from build123d import *

# Parameters (mm, degrees)
SKETCH1_W             = 2
SKETCH1_H             = 2
SKETCH1_W_2           = 21
SKETCH1_H_2           = 15
SKETCH1_H_3           = 1
IMU_BASE_DEPTH        = 7
SCREW_CHANNELS_DEPTH  = 14
SKETCH1_13_W          = 2
SKETCH1_13_H          = 1
NUT_CHANNELS_DEPTH    = 3
SKETCH2_W             = 23
SKETCH2_H             = 15
SOLDER_CHANNELS_DEPTH = 2.5
IMU_EXTENSION_DEPTH   = 15


with BuildPart() as part:
    # Sketch1 → IMU_Base (new body)
    with BuildSketch(Plane.XY):
        Polygon((-2, 0), (0, 0), (0, 1), (0, 5), (0, 6), (0, 21), (0, 21.55806344), (0, 22), (0, 26), (0, 27), (0.75, 27), (5.75, 27), (6.5, 27), (14.5, 27), (15.25, 27), (20.25, 27), (21, 27), (23, 27), (23, 29), (-2, 29), align=None)
        Polygon((0.75, 0), (0, 0), (0, -2), (23, -2), (23, 0), (21, 0), (20.25, 0), (15.25, 0), (14.5, 0), (6.5, 0), (5.75, 0), align=None)
        with Locations((-1, -1)):
            Rectangle(SKETCH1_W, SKETCH1_H)
        with Locations((10.5, 13.5)):
            Rectangle(SKETCH1_W_2, SKETCH1_H_2)
        with Locations((22, 13.5)):
            Rectangle(SKETCH1_W, SKETCH1_H_2)
        Polygon((21, 22), (21, 21), (23, 21), (23, 21.848888028), (23, 22), align=None)
        Polygon((0, 21.55806344), (0, 21), (21, 21), (21, 22), (18.5, 22), (2.5, 22), (0, 22), align=None)
        Polygon((23, 26), (23, 27), (21, 27), (20.25, 27), (15.25, 27), (14.5, 27), (6.5, 27), (5.75, 27), (0.75, 27), (0, 27), (0, 26), (2.5, 26), (18.5, 26), (21, 26), align=None)
        with BuildLine():
            Line((23, 22), (23, 26))
            Line((23, 26), (21, 26))
            Line((21, 26), (18.5, 26))
            Line((18.5, 26), (2.5, 26))
            ThreePointArc((2.5, 26), (0.5, 24), (2.5, 22))
            Line((2.5, 22), (18.5, 22))
            Line((18.5, 22), (21, 22))
            Line((21, 22), (23, 22))
        make_face()
        with BuildLine():
            Line((0, 26), (0, 22))
            Line((0, 22), (2.5, 22))
            ThreePointArc((2.5, 22), (0.5, 24), (2.5, 26))
            Line((2.5, 26), (0, 26))
        make_face()
        Polygon((0, 6), (0, 5), (2.5, 5), (18.5, 5), (21, 5), (21, 6), align=None)
        with Locations((22, 5.5)):
            Rectangle(SKETCH1_W, SKETCH1_H_3)
        with BuildLine():
            ThreePointArc((2.5, 5), (0.5, 3), (2.5, 1))
            Line((2.5, 1), (18.5, 1))
            Line((18.5, 1), (21, 1))
            Line((21, 1), (23, 1))
            Line((23, 1), (23, 5))
            Line((23, 5), (21, 5))
            Line((21, 5), (18.5, 5))
            Line((18.5, 5), (2.5, 5))
        make_face()
        with BuildLine():
            Line((0, 5), (0, 1))
            Line((0, 1), (2.5, 1))
            ThreePointArc((2.5, 1), (0.5, 3), (2.5, 5))
            Line((2.5, 5), (0, 5))
        make_face()
        Polygon((0, 1), (0, 0), (0.75, 0), (5.75, 0), (6.5, 0), (14.5, 0), (15.25, 0), (20.25, 0), (21, 0), (21, 1), (18.5, 1), (2.5, 1), align=None)
        with Locations((22, 0.5)):
            Rectangle(SKETCH1_W, SKETCH1_H_3)
    extrude(amount=IMU_BASE_DEPTH)

    # Sketch1_12 → Screw_Channels (cut)
    with BuildSketch(Plane.XY):
        with BuildLine():
            Line((23, 22), (23, 26))
            Line((23, 26), (21, 26))
            Line((21, 26), (18.5, 26))
            Line((18.5, 26), (2.5, 26))
            ThreePointArc((2.5, 26), (0.5, 24), (2.5, 22))
            Line((2.5, 22), (18.5, 22))
            Line((18.5, 22), (21, 22))
            Line((21, 22), (23, 22))
        make_face()
        with BuildLine():
            ThreePointArc((2.5, 5), (0.5, 3), (2.5, 1))
            Line((2.5, 1), (18.5, 1))
            Line((18.5, 1), (21, 1))
            Line((21, 1), (23, 1))
            Line((23, 1), (23, 5))
            Line((23, 5), (21, 5))
            Line((21, 5), (18.5, 5))
            Line((18.5, 5), (2.5, 5))
        make_face()
    extrude(amount=SCREW_CHANNELS_DEPTH, mode=Mode.SUBTRACT)

    # Sketch1_13 → Nut_Channels (cut)
    with BuildSketch(Plane.XY):
        Polygon((23, 26), (23, 27), (21, 27), (20.25, 27), (15.25, 27), (14.5, 27), (6.5, 27), (5.75, 27), (0.75, 27), (0, 27), (0, 26), (2.5, 26), (18.5, 26), (21, 26), align=None)
        with BuildLine():
            Line((0, 26), (0, 22))
            Line((0, 22), (2.5, 22))
            ThreePointArc((2.5, 22), (0.5, 24), (2.5, 26))
            Line((2.5, 26), (0, 26))
        make_face()
        Polygon((0, 21.55806344), (0, 21), (21, 21), (21, 22), (18.5, 22), (2.5, 22), (0, 22), align=None)
        Polygon((21, 22), (21, 21), (23, 21), (23, 21.848888028), (23, 22), align=None)
        with Locations((22, 5.5)):
            Rectangle(SKETCH1_13_W, SKETCH1_13_H)
        Polygon((0, 6), (0, 5), (2.5, 5), (18.5, 5), (21, 5), (21, 6), align=None)
        with Locations((22, 0.5)):
            Rectangle(SKETCH1_13_W, SKETCH1_13_H)
        Polygon((0, 1), (0, 0), (0.75, 0), (5.75, 0), (6.5, 0), (14.5, 0), (15.25, 0), (20.25, 0), (21, 0), (21, 1), (18.5, 1), (2.5, 1), align=None)
        with BuildLine():
            Line((0, 5), (0, 1))
            Line((0, 1), (2.5, 1))
            ThreePointArc((2.5, 1), (0.5, 3), (2.5, 5))
            Line((2.5, 5), (0, 5))
        make_face()
    extrude(amount=NUT_CHANNELS_DEPTH, mode=Mode.SUBTRACT)

    # Sketch2 → Solder_Channels (cut)
    with BuildSketch(Plane.XY.offset(7)):
        with Locations((11.5, 13.5)):
            Rectangle(SKETCH2_W, SKETCH2_H)
    extrude(amount=-SOLDER_CHANNELS_DEPTH, mode=Mode.SUBTRACT)

    # Sketch4 → IMU_Extension (add)
    with BuildSketch(Plane(origin=(23, 0, 0), x_dir=(0, 0, -1), z_dir=(1, 0, 0))):
        Polygon((-7, 26), (-7, 29), (0, 29), (0, 27), (-3, 27), (-3, 26), align=None)
        Polygon((-7, 22), (-3, 22), (-3, 21), (0, 21), (0, 6), (-3, 6), (-3, 5), (-7, 5), (-7, 6), (-4.5, 6), (-4.5, 21), (-7, 21), align=None)
        Polygon((-7, 1), (-3, 1), (-3, 0), (0, 0), (0, -2), (-7, -2), align=None)
    extrude(amount=IMU_EXTENSION_DEPTH)


solid = part.part
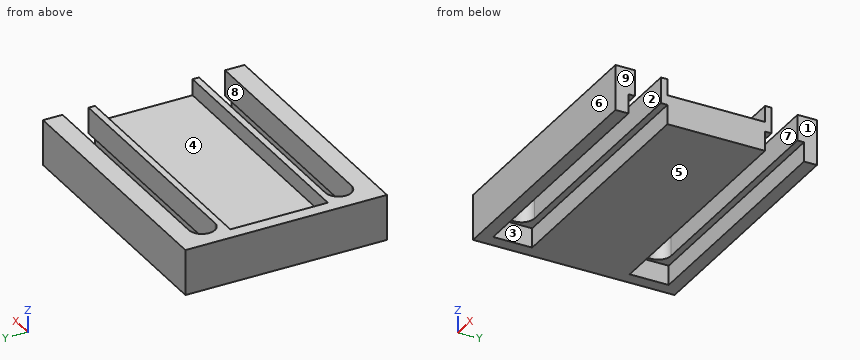
Geometry check sheet. Reference: the model listing, model coordinates, mm. Face numbers are marked on the shaded views. A direction names the side the tool comes from. Give positions to 0.01 mm unless a question says otherwise; leave off trailing zeros. Loops run counter-clockwise (first coordinate to the right, second up) from the corner with the lowest first, then second, coordinate; pieces in that order, holes last. Notation, with made-up numbers: M 67.25,36 L 79.25,36 A26 ccw 79.25,73 Z; hole C 4,28.5 d4. An arc over 180 degrees is marked long. Answer as a JSON object with one key per item and string values. Group by question number.
Item 1: Sectioned sample at C-C on y = 3. Record the boundary of the cut face in (x, z).
Item 2: Access from +Z, -Z, +X, -X, +Y, -Y to the whole of each face (thin tool, end or side, straight path). Record for the marked faces 1, 2, 3, 4 and 5.
Item 3: Sectioned sample at D-D on y = 19. Record the boundary of the cut face in (x, z), plus the area to 3 significant figures.
Item 4: Gauge pin test, flat ends, axial feed: pin 1 (12 mm diameter, centred on x = 16.5, y = 13.5, fed in from +Z); pin 2 (3 mm diameter, centred on y = 13, z = 5, fed in from +X); pin 3 (1.5 mm diameter, centred on y = 24, z = 1, fed in from +X). Record the tip position at first contact, or that the pin passes through.
Item 5: Material ranges on L1, parallel to Y at x = 35, z = 6; L2, parallel to Y at x = 4, z = 2; L3, parallel to Y at x = 24, z = 4, recorded low to high.
Item 6: Mould release check, pull along Y, two halves, no side actions. Record for the marked faces 6, 7, 8 and 9: pulls with the +Y half, pulls with the -Y half, needs draft (parallel to the pull), parting line crosses it, or undercut.
Item 7: Sectioned sample at B-B on z = 6. Record the boundary of the cut face in (x, y), plus the area to 3 significant figures.
Item 8: Sectioned sample at A-A on x = 26.5. Record the boundary of the cut face in (y, z), plus the area to 4 significant figures.
Findings below:
{
 "1": {"outline": "M -2,0 L 0,0 L 0,3 L 0.5,3 L 0.5,7 L -2,7 Z"},
 "2": {"face 1": "+Z, -Z, +X, +Y, -Y", "face 2": "+Z, -Z, +X", "face 3": "-Z, +X", "face 4": "+Z, +X", "face 5": "-Z, +X, -X, +Y, -Y"},
 "3": {"outline": "M -2,0 L 38,0 L 38,4.5 L 0,4.5 L 0,7 L -2,7 Z", "area": "185 mm2"},
 "4": {"pin 1": "z = 4.5", "pin 2": "x = 38", "pin 3": "x = 0"},
 "5": {"L1": "-2 to 1, 5 to 6, 21 to 22, 26 to 29", "L2": "-2 to 0, 6 to 21, 27 to 29", "L3": "-2 to 1, 5 to 22, 26 to 29"},
 "6": {"face 6": "pulls with the -Y half", "face 7": "undercut", "face 8": "undercut", "face 9": "needs draft"},
 "7": {"outline": "M -2,-2 L 38,-2 L 38,1 L 2.5,1 A2 cw 2.5,5 L 38,5 L 38,6 L 0,6 L 0,21 L 38,21 L 38,22 L 2.5,22 A2 cw 2.5,26 L 38,26 L 38,29 L -2,29 Z", "area": "373 mm2"},
 "8": {"outline": "M -2,0 L 0,0 L 0,3 L 1,3 L 1,7 L -2,7 Z; M 5,3 L 6,3 L 6,0 L 21,0 L 21,3 L 22,3 L 22,7 L 21,7 L 21,4.5 L 6,4.5 L 6,7 L 5,7 Z; M 26,3 L 27,3 L 27,0 L 29,0 L 29,7 L 26,7 Z", "area": "111.5 mm2"}
}
